Source: CAD feature listing. Evaluate the final solid. Frame: model axes, mm. A direction names the side the tool comes from. Give positions to 0.01 mm unless a question says otherwise; leave off trailing zeros. Write each loop counter-clockwise with the first axis right and the second up, starting at its lowest first coordinate (ties: lowest second). Pieces come first, ordered by that corner, then holes.
```python
from build123d import *

# Parameters (mm, degrees)
F0_W     = 688.975
F0_H     = 44.45
F1_DEPTH = 15.875
F2_W     = 15.875
F2_H     = 22.225
F3_DEPTH = 15.876


with BuildPart() as f1:
    # F0 (on Front) → F1 (new body)
    with BuildSketch(Plane.XZ):
        Rectangle(F0_W, F0_H)
    extrude(amount=F1_DEPTH)

    # F2 (on face) → F3 (cut, through all)
    with BuildSketch(Plane.XZ):
        with Locations((-336.55, -11.1125)):
            Rectangle(F2_W, F2_H)
        with Locations((336.55, -11.1125)):
            Rectangle(F2_W, F2_H)
    extrude(amount=F3_DEPTH, mode=Mode.SUBTRACT)


solid = f1.part
```
1. Cut plane A-A, the plane y = -7. Return the cut outline in (x, z) (1 decimal), then the cut area to 3 significant figures.
2. Contact query for flat-ended pins moving along their axis: P1, Ø1, axis at y = -1.5, z = -15.5, coming from the +X side; P2, Ø6, axis at x = -25.5, z = -3, coming from the +Y side. Output: stop coordinate, or through.
3. Access query for faces 1 (the flat face through (328.612, -8, -11)), 2 (the flat face through (-337, -8, 0)), 3 (the flat face through (-5, -8, -22.225)). Directions: +Z, -Z, +X, -X, +Y, -Y. A direction counts if a zero-diameter tool reaches every point of the face in a straight line with its end or side. Return the directions, or none.
4. Cut plane B-B, the plane z = -13.5. Return the cut outline in (x, y) (1 decimal), then the cut area to 3 significant figures.
5. Line query: L1, parallel to X at y = -3, z = -4. Output: solid intervals per line, ascending.
Response values:
1. outline: (-344.5, 0) - (-328.6, 0) - (-328.6, -22.2) - (328.6, -22.2) - (328.6, 0) - (344.5, 0) - (344.5, 22.2) - (-344.5, 22.2) - close
1. area: 29,900 mm2
2. P1: stops at x = 328.61
2. P2: stops at y = 0
3. face 1: -Z, +X, +Y, -Y
3. face 2: -Z, -X, +Y, -Y
3. face 3: -Z, +X, -X, +Y, -Y
4. outline: (-328.6, -15.9) - (328.6, -15.9) - (328.6, 0) - (-328.6, 0) - close
4. area: 10,400 mm2
5. L1: x = -328.61 to 328.61
